```python
from build123d import *

# Parameters (mm, degrees)
F1_DEPTH = 40
F2_W     = 174
F2_H     = 64
F3_DEPTH = 2


with BuildPart() as f1:
    # F0 (on Top) → F1 (new body)
    with BuildSketch(Plane.XY):
        with BuildLine():
            Line((0, 64), (0, 0))
            Line((0, 0), (12.5, 0))
            Line((12.5, 0), (12.5, 2))
            Line((12.5, 2), (5, 2))
            Line((5, 2), (5, 29))
            Line((5, 29), (35, 29))
            Line((35, 29), (35, 2))
            Line((35, 2), (27.5, 2))
            Line((27.5, 2), (27.5, 0))
            Line((27.5, 0), (47.5, 0))
            Line((47.5, 0), (47.5, 2))
            Line((47.5, 2), (40, 2))
            Line((40, 2), (40, 29))
            Line((40, 29), (70, 29))
            Line((70, 29), (70, 2))
            Line((70, 2), (62.5, 2))
            Line((62.5, 2), (62.5, 0))
            Line((62.5, 0), (86, 0))
            Line((86, 0), (86, 2))
            Line((86, 2), (85, 2))
            Line((85, 2), (85, 21))
            Line((85, 21), (102, 21))
            Line((102, 21), (102, 2))
            Line((102, 2), (101, 2))
            Line((101, 2), (101, 0))
            Line((101, 0), (121, 0))
            Line((121, 0), (121, 2))
            Line((121, 2), (117, 2))
            Line((117, 2), (121, 8.9282032303))
            Line((121, 8.9282032303), (128.5, 21.918584287))
            Line((128.5, 21.918584287), (136, 8.9282032303))
            Line((136, 8.9282032303), (140, 2))
            Line((140, 2), (136, 2))
            Line((136, 2), (136, 0))
            Line((136, 0), (149, 0))
            Line((149, 0), (149, 2))
            Line((149, 2), (145, 2))
            Line((145, 2), (149, 8.9282032303))
            Line((149, 8.9282032303), (156.5, 21.918584287))
            Line((156.5, 21.918584287), (164, 8.9282032303))
            Line((164, 8.9282032303), (168, 2))
            Line((168, 2), (164, 2))
            Line((164, 2), (164, 0))
            Line((164, 0), (174, 0))
            Line((174, 0), (174, 64))
            Line((174, 64), (166, 64))
            Line((166, 64), (166, 60.8484692283))
            ThreePointArc((166, 60.8484692283), (168.2211110476, 57.4686269666), (169, 53.5))
            ThreePointArc((169, 53.5), (154.5313730334, 43.7788889524), (151, 60.8484692283))
            Line((151, 60.8484692283), (151, 64))
            Line((151, 64), (140, 64))
            Line((140, 64), (140, 60.8484692283))
            ThreePointArc((140, 60.8484692283), (142.2211110476, 57.4686269666), (143, 53.5))
            ThreePointArc((143, 53.5), (128.5313730334, 43.7788889524), (125, 60.8484692283))
            Line((125, 60.8484692283), (125, 64))
            Line((125, 64), (112, 64))
            Line((112, 64), (112, 61.5))
            ThreePointArc((112, 61.5), (115.6803398875, 57.0901699437), (117, 51.5))
            ThreePointArc((117, 51.5), (98.9098300563, 40.3196601125), (97, 61.5))
            Line((97, 61.5), (97, 64))
            Line((97, 64), (82, 64))
            Line((82, 64), (82, 61.5))
            ThreePointArc((82, 61.5), (85.6803398875, 57.0901699437), (87, 51.5))
            ThreePointArc((87, 51.5), (68.9098300563, 40.3196601125), (67, 61.5))
            Line((67, 61.5), (67, 64))
            Line((67, 64), (52, 64))
            Line((52, 64), (52, 61.5))
            ThreePointArc((52, 61.5), (55.6803398875, 57.0901699437), (57, 51.5))
            ThreePointArc((57, 51.5), (38.9098300563, 40.3196601125), (37, 61.5))
            Line((37, 61.5), (37, 64))
            Line((37, 64), (25, 64))
            Line((25, 64), (25, 61.5))
            ThreePointArc((25, 61.5), (28.6803398875, 57.0901699437), (30, 51.5))
            ThreePointArc((30, 51.5), (11.9098300563, 40.3196601125), (10, 61.5))
            Line((10, 61.5), (10, 64))
            Line((10, 64), (0, 64))
        make_face()
    extrude(amount=F1_DEPTH)

    # F2 (on face) → F3 (join)
    with BuildSketch(Plane(origin=(0, 0, 0), x_dir=(1, 0, 0), z_dir=(0, 0, -1))):
        with Locations((87, -32)):
            Rectangle(F2_W, F2_H)
    extrude(amount=F3_DEPTH)


solid = f1.part
```
Can you work these out from the model? Positions are in its coordinate system, mm. A direction names the side the tool comes from. Coordinates: 2 decimals unless noted, no trailing zeros. Write each loop counter-clockwise with the first axis right and the second up, starting at its lowest first coordinate (ties: lowest second). Pieces come first, ordered by that corner, then holes. Notation, with made-up numbers: M -39,-1.75 L 14,-1.75 A14 cw 14,9.25 Z; hole C 35.25,82 d7. An arc over 180 degrees is marked long. Answer as CSV lines item,"result".
Item 1: Imagine slicing it at D-D on y = 49. List the corners of the cut face in (x, z) for me, plus the area to 3 significant figures.
Geometry results:
outline,"M 0,-2 L 174,-2 L 174,40 L 167.99,40 L 167.99,0 L 149.01,0 L 149.01,40 L 141.99,40 L 141.99,0 L 123.01,0 L 123.01,40 L 116.75,40 L 116.75,0 L 92.25,0 L 92.25,40 L 86.75,40 L 86.75,0 L 62.25,0 L 62.25,40 L 56.75,40 L 56.75,0 L 32.25,0 L 32.25,40 L 29.75,40 L 29.75,0 L 5.25,0 L 5.25,40 L 0,40 Z"
area,"1,870 mm2"
Item 2: We'd pull the mould along Y, two halves only. Please class faces 4 (the flat face through (138, 2, 20)), 5 (the flat face through (125, 62, 20)), 6 (the flat face through (66, 0, 19)): +Y half, -Y half, draft (parallel to the pull), parting line (faces both ways), or undercut.
Geometry results:
face 4,"undercut"
face 5,"draft"
face 6,"-Y half"
Item 3: I'm going to push flat-ended pins straight in: P1, Ø12.5, axis at x = 132.5, y = 53.5, coming from the +Z side; P2, Ø1, axis at x = 41.5, z = 5.5, coming from the +Y side; P3, Ø0.5, axis at x = 101.5, z = 25.5, coming from the +Y side. Where does each tip first touch, or does it pass through?
Geometry results:
P1,"stops at z = 0"
P2,"stops at y = 39.5"
P3,"stops at y = 39.43"
Item 4: Imagine slicing it at A-A on x = 17.5. List the corners of the cut face in (y, z) for me.
Geometry results:
outline,"M 0,-2 L 64,-2 L 64,0 L 39,0 L 39,40 L 29,40 L 29,0 L 0,0 Z"
Item 5: Imagine slicing it at B-B on y = 26.5. List the corners of the cut face in (x, z) for me.
Geometry results:
outline,"M 0,-2 L 174,-2 L 174,40 L 70,40 L 70,0 L 40,0 L 40,40 L 35,40 L 35,0 L 5,0 L 5,40 L 0,40 Z"
Item 6: Please list where these lines run through material, in increasing order: line 1 along X through (y, z) = (16.5, 33); line 2 along X through (y, z) = (20, 31.5); line 3 along Y through (x, z) = (31, 15).
Geometry results:
line 1,"x = 0 to 5, 35 to 40, 70 to 85, 102 to 125.37, 131.63 to 153.37, 159.63 to 174"
line 2,"x = 0 to 5, 35 to 40, 70 to 85, 102 to 127.39, 129.61 to 155.39, 157.61 to 174"
line 3,"y = 0 to 2, 29 to 64"
Item 7: On a 3-axis mill with a long thin cutter (end or side, diameter ignored), from which of +Z, -Z, +X, -X, +Y, -Y can I reach the whole of each face in a straight line? I mean faces 1 (the flat face through (140, 62, 20)), 2 (the flat face through (105, 32, 40)), 3 (the flat face through (55, 29, 20)). Say none if no direction works.
Geometry results:
face 1,"+Z, +Y"
face 2,"+Z, +X, -X, +Y, -Y"
face 3,"+Z"
Item 8: Imagine slicing it at C-C on x = 44.5. List the corners of the cut face in (y, z) for me.
Geometry results:
outline,"M 0,-2 L 64,-2 L 64,0 L 39,0 L 39,40 L 29,40 L 29,0 L 2,0 L 2,40 L 0,40 Z"
